Source: CAD feature listing. Evaluate the final solid. Frame: model axes, mm. Face numbers are marked on the shaded views. A direction names the side the tool comes from. Give positions to 0.01 mm unless a question says otherwise; leave off trailing zeros. Order: outer loops, then holes, each group sorted by start corner. A loop starts at its lowest first (then second) coordinate and runs counter-clockwise, first axis right, second up. Notation, with made-up numbers: M 54,-10.5 L 65,-10.5 A28 cw 65,9.5 Z; hole C 38,-23.5 d10. An arc over 180 degrees is marked long. One line per question, with ' | ' between items. Start each with the question number.
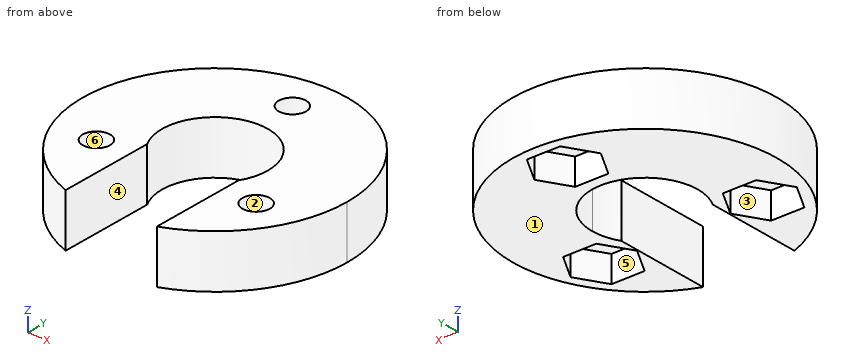
from build123d import *

# Parameters (mm, degrees)
F1_DEPTH = 6
F2_START = 3
F0_R     = 1.55
F2_DEPTH = 3


with BuildPart() as f1:
    # F0 (on Top) → F1 (new body)
    with BuildSketch(Plane.XY):
        with BuildLine():
            ThreePointArc((-5.2, -2.9933259094), (-1.5491933385, 5.7965506985), (6, 0))
            ThreePointArc((6, 0), (5.7965506985, -1.5491933385), (5.2, -2.9933259094))
            Line((5.2, -2.9933259094), (5.2, -14.0698258696))
            ThreePointArc((5.2, -14.0698258696), (12.3085336251, -8.5732140997), (15, 0))
            ThreePointArc((15, 0), (-8.5732140997, 12.3085336251), (-5.2, -14.0698258696))
            Line((-5.2, -14.0698258696), (-5.2, -2.9933259094))
        make_face()
        Polygon((-10.9840888713, -8.525), (-12.8749110029, -5.25), (-10.9840888713, -1.975), (-7.2024446081, -1.975), (-5.3116224765, -5.25), (-7.2024446081, -8.525), align=None, mode=Mode.SUBTRACT)
        Polygon((12.8749110029, -5.25), (10.9840888713, -8.525), (7.2024446081, -8.525), (5.3116224765, -5.25), (7.2024446081, -1.975), (10.9840888713, -1.975), align=None, mode=Mode.SUBTRACT)
        Polygon((3.7816442632, 10.5), (1.8908221316, 7.225), (-1.8908221316, 7.225), (-3.7816442632, 10.5), (-1.8908221316, 13.775), (1.8908221316, 13.775), align=None, mode=Mode.SUBTRACT)
    extrude(amount=F1_DEPTH)

    # F0 (on Top) → F2 (join)
    with BuildSketch(Plane.XY.offset(F2_START)):
        Polygon((7.2024446081, -8.525), (10.9840888713, -8.525), (12.8749110029, -5.25), (10.9840888713, -1.975), (7.2024446081, -1.975), (5.3116224765, -5.25), align=None)
        with Locations((9.0932667397, -5.25)):
            Circle(F0_R, mode=Mode.SUBTRACT)
        Polygon((-1.8908221316, 7.225), (1.8908221316, 7.225), (3.7816442632, 10.5), (1.8908221316, 13.775), (-1.8908221316, 13.775), (-3.7816442632, 10.5), align=None)
        with Locations((0, 10.5)):
            Circle(F0_R, mode=Mode.SUBTRACT)
        Polygon((-10.9840888713, -1.975), (-12.8749110029, -5.25), (-10.9840888713, -8.525), (-7.2024446081, -8.525), (-5.3116224765, -5.25), (-7.2024446081, -1.975), align=None)
        with Locations((-9.0932667397, -5.25)):
            Circle(F0_R, mode=Mode.SUBTRACT)
    extrude(amount=F2_DEPTH)


solid = f1.part
Item 1: Reachability of the marked faces 4, 5 and 6 from +Z, -Z, +X, -X, +Y, -Y: full face, straight path, thin tool, end or side. Return the list, or none.
Item 2: Cut plane A-A on x = 0. Return the cut outline in (y, z) (3 decimals).
Item 3: Pin query (flat end, axial travel): pin 1 Ø11 at (x, y) = (0, 0) entering from +Z; pin 2 Ø7 at (x, y) = (-0.5, 10) entering from -Z; pin 3 Ø1.5 at (x, z) = (0, 2) entering from -Y; pin 4 Ø3.5 at (x, z) = (-9, 1) entering from -Y. Return the tip coordinate at first contact, or that it passes through.
Item 4: Cut plane C-C on y = 2.75. Return the cut outline in (x, z).
Item 5: Cut plane D-D on z = 1.25. Return the cut outline in (x, y) (3 decimals), and give its area (3 significant figures).
Item 6: Cut plane B-B on z = 4. Return the cut outline in (x, y).
Item 7: Mould query, pull axis Y, two halves, no side actions, for the marked faces 1, 2 and 3. Classes: pulls with the +Y half, pulls with the -Y half, needs draft (parallel to the pull), parting line crosses it, or undercut.
Item 8: Line query: line 1 (Y direction, x = 0, z = 3.9); line 2 (Y direction, x = -10, z = 3.55); line 3 (X direction, y = -11.75, z = 3.05). Output: solid intervals per line, ascending.
Results are:
1) face 4: +Z, -Z, -Y | face 5: -Z | face 6: +Z, -Z
2) outline: M 6,0 L 7.225,0 L 7.225,3 L 8.95,3 L 8.95,6 L 6,6 Z; M 12.05,3 L 13.775,3 L 13.775,0 L 15,0 L 15,6 L 12.05,6 Z
3) pin 1: passes through | pin 2: stops at z = 0 | pin 3: stops at y = 5.95 | pin 4: stops at y = -13.13
4) outline: M -14.75,0 L -5.33,0 L -5.33,6 L -14.75,6 Z; M 5.33,0 L 14.75,0 L 14.75,6 L 5.33,6 Z
5) outline: M -5.2,-14.07 L -5.2,-2.993 A6 cw long 5.2,-2.993 L 5.2,-14.07 A15 ccw long Z; hole M -12.875,-5.25 L -10.984,-8.525 L -7.202,-8.525 L -5.312,-5.25 L -7.202,-1.975 L -10.984,-1.975 Z; hole M -3.782,10.5 L -1.891,7.225 L 1.891,7.225 L 3.782,10.5 L 1.891,13.775 L -1.891,13.775 Z; hole M 5.312,-5.25 L 7.202,-8.525 L 10.984,-8.525 L 12.875,-5.25 L 10.984,-1.975 L 7.202,-1.975 Z | area: 383 mm2
6) outline: M -5.2,-14.07 L -5.2,-2.99 A6 cw long 5.2,-2.99 L 5.2,-14.07 A15 ccw long Z; hole C -9.09,-5.25 d3.1; hole C 0,10.5 d3.1; hole C 9.09,-5.25 d3.1
7) face 1: needs draft | face 2: undercut | face 3: undercut
8) line 1: y = 6 to 8.95, 12.05 to 15 | line 2: y = -11.18 to -6.51, -3.99 to 11.18 | line 3: x = -9.32 to -5.2, 5.2 to 9.32
